from build123d import *

# Parameters (mm, degrees)
F0_W     = 66.548
F0_H     = 25.273
F1_DEPTH = 3.175
F2_W     = 66.548
F2_H     = 25.273
F2_W_2   = 63.373
F2_H_2   = 22.098
F3_DEPTH = 15.875
F4_W     = 1.5875
F4_H     = 22.098
F5_DEPTH = 3.048
F6_W     = 22.098
F6_H     = 1.5875
F7_DEPTH = 3.175
F8_W     = 1.5875
F8_H     = 22.098
F9_DEPTH = 1.5875


with BuildPart() as f1:
    # F0 (on Top) → F1 (new body)
    with BuildSketch(Plane.XY):
        with Locations((33.274, -12.6365)):
            Rectangle(F0_W, F0_H)
    extrude(amount=F1_DEPTH)

    # F2 (on face) → F3 (join)
    with BuildSketch(Plane.XY.offset(3.175)):
        with Locations((33.274, -12.6365)):
            Rectangle(F2_W, F2_H)
        with Locations((33.274, -12.6365)):
            Rectangle(F2_W_2, F2_H_2, mode=Mode.SUBTRACT)
    extrude(amount=F3_DEPTH)

    # F4 (on face) → F5 (join)
    with BuildSketch(Plane.XY.offset(19.05)):
        with Locations((65.75425, -12.6365)):
            Rectangle(F4_W, F4_H)
    extrude(amount=F5_DEPTH)

    # F6 (on face) → F7 (join)
    with BuildSketch(Plane.YZ.offset(66.548)):
        with Locations((-12.6365, 18.25625)):
            Rectangle(F6_W, F6_H)
    extrude(amount=F7_DEPTH)

    # F8 (on face) → F9 (join)
    with BuildSketch(Plane(origin=(0, 0, 17.4625), x_dir=(1, 0, 0), z_dir=(0, 0, -1))):
        with Locations((68.92925, 12.6365)):
            Rectangle(F8_W, F8_H)
    extrude(amount=F9_DEPTH)


solid = f1.part
Source: CAD feature listing. Evaluate the final solid. Frame: model axes, mm. A direction names the side the tool comes from. Round coordinates to 2 decimals unless told otherwise and drop trailing zeros. Order: outer loops, then holes, each group sorted by start corner. A loop starts at its lowest first (then second) coordinate and runs counter-clockwise, first axis right, second up. Notation, with made-up numbers: (40, -6.75) - (92, -6.75) arc R28 cw to (92, 19.25) - close; hole circle Ø6 at (45, 10.25). An arc over 180 degrees is marked (long way). Use a Markdown table: item, result. Add a question column.
1. Line query: probe 1 along X at (y, z) = (-6, 16.25); probe 2 along Y at (x, z) = (60.5, 5.75); probe 3 along X at (y, z) = (-7.25, 19). Output: solid intervals per line, ascending.
2. Section query B-B (z = 13.5). Return the cut outline in (x, y).
3. Section query A-A (z = 16.75). Return the cut outline in (x, y).
4. Set-up query: faces 4 (the flat face through (68, -1.588, 18)), 5 (the flat face through (69, -13, 15.875)), 6 (the flat face through (66, -1.588, 21)), 7 (the flat face through (33, -12, 3.175)). Return all of +Z, -Z, +X, -X, +Y, -Y with unobstructed straight access to the full face (end or side cutting, diameter ignored); none if empty.
5. First-contact query: pin 1 (1.5 mm diameter, centred on x = 51.5, y = -17, fed in from +Z) (3 decimals); pin 2 (2.5 mm diameter, centred on x = 69, y = -10.5, fed in from +Z); pin 3 (0.5 mm diameter, centred on x = 69, y = -14, fed in from -Z) (3 decimals). Flat tips, straight axial feed; report the tip coordinate or a pass-through.
6. Mould query, pull axis X, two halves, no side actions, for faces 1 (the flat face through (69.723, -12, 17)), 2 (the flat face through (66, -12, 22.098)), 3 (the flat face through (68.136, -12, 17)). Classes: +X half, -X half, draft (parallel to the pull), parting line (faces both ways), or undercut.
Derived:
| question | item | result |
|---|---|---|
| 1 | probe 1 | 0 to 1.59, 64.96 to 66.55, 68.14 to 69.72 |
| 1 | probe 2 | -25.27 to -23.69, -1.59 to 0 |
| 1 | probe 3 | 0 to 1.59, 64.96 to 69.72 |
| 2 | outline | (0, -25.27) - (66.55, -25.27) - (66.55, 0) - (0, 0) - close; hole (1.59, -23.69) - (64.96, -23.69) - (64.96, -1.59) - (1.59, -1.59) - close |
| 3 | outline | (0, -25.27) - (66.55, -25.27) - (66.55, 0) - (0, 0) - close; (68.14, -23.69) - (69.72, -23.69) - (69.72, -1.59) - (68.14, -1.59) - close; hole (1.59, -23.69) - (64.96, -23.69) - (64.96, -1.59) - (1.59, -1.59) - close |
| 4 | face 4 | +Z, -Z, +X, +Y |
| 4 | face 5 | -Z, +X, +Y, -Y |
| 4 | face 6 | +Z, +X, -X, +Y |
| 4 | face 7 | +Z |
| 5 | pin 1 | z = 3.175 |
| 5 | pin 2 | z = 19.05 |
| 5 | pin 3 | z = 15.875 |
| 6 | face 1 | +X half |
| 6 | face 2 | draft |
| 6 | face 3 | undercut |
